Verification items for the finished model (mm, model axes). A direction names the side the tool comes from. Round coordinates to 2 decimals unless told otherwise and drop trailing zeros. Write each loop counter-clockwise with the first axis right and the second up, starting at its lowest first coordinate (ties: lowest second). Pieces come first, ordered by that corner, then holes.
from build123d import *

# Parameters (mm, degrees)
SKETCH1_W           = 16
SKETCH1_H           = 32
SKETCH1_R           = 1.5
SKETCH1_W_2         = 8
SKETCH1_H_2         = 150
BOSS_EXTRUDE1_DEPTH = 6.35
FILLET1_R           = 10
FILLET2_R           = 10
CHAMFER1_SIZE       = 10
SKETCH2_R           = 1.65
CUT_EXTRUDE1_DEPTH  = 10


with BuildPart() as part:
    # Sketch1 → Boss-Extrude1 (new body)
    # profile 1 of 3: a face of its own
    with BuildSketch(Plane.XY):
        Rectangle(SKETCH1_W, SKETCH1_H)
        with Locations((0, -8)):
            Circle(SKETCH1_R, mode=Mode.SUBTRACT)
        with Locations((0, 8)):
            Circle(SKETCH1_R, mode=Mode.SUBTRACT)
        Circle(SKETCH1_R, mode=Mode.SUBTRACT)
    # profile 2 of 3: a face of its own
    with BuildSketch(Plane.XY):
        with Locations((-4, 91)):
            Rectangle(SKETCH1_W_2, SKETCH1_H_2)
    # profile 3 of 3: a face of its own
    with BuildSketch(Plane.XY):
        Polygon((-23, -16), (-23, 166), (-8, 166), (-8, 16), (-8, -16), align=None)
    extrude(amount=BOSS_EXTRUDE1_DEPTH)

    # Fillet1
    # the kernel refuses this fillet: 10 mm, written as the material it adds along each edge
    with BuildSketch(Plane(origin=(0, 16, 0), x_dir=(0, 1, 0), z_dir=(0, 0, 1))) as fillet1_piece_1:
        with BuildLine():
            CenterArc((9.797958971, -10), FILLET1_R, 90, 78.463040967)
            Line((0, -8), (0, 0))
            Line((0, 0), (9.797958971, 0))
        make_face()
    extrude(amount=6.35)
    # the kernel refuses this fillet: 10 mm, written as the material it takes off along each edge
    with BuildSketch(Plane(origin=(8, -16, -25), x_dir=(0, 1, 0), z_dir=(0, 0, 1)), Plane(origin=(-23, -16, -25), x_dir=(1, 0, 0), z_dir=(0, 0, 1))) as fillet1_2_piece_1:
        with BuildLine():
            CenterArc((FILLET1_R, FILLET1_R), FILLET1_R, 180, 90)
            Line((0, FILLET1_R), (0, 0))
            Line((0, 0), (FILLET1_R, 0))
        make_face()
    extrude(amount=56.35, mode=Mode.SUBTRACT)

    # Fillet2
    fillet2_edges = [part.edges().sort_by_distance(p)[0] for p in [
        (8, 16, 3.175),
    ]]
    fillet(fillet2_edges, radius=FILLET2_R)

    # Chamfer1
    chamfer1_edges = [part.edges().sort_by_distance(p)[0] for p in [
        (-23, 166, 3.175),
    ]]
    chamfer(chamfer1_edges, length=CHAMFER1_SIZE)

    # Sketch2 → Cut-Extrude1 (cut)
    with BuildSketch(Plane.XY.offset(6.35)):
        with Locations((-13, 156)):
            Circle(SKETCH2_R)
        with Locations((-13, 106)):
            Circle(SKETCH2_R)
    extrude(amount=-CUT_EXTRUDE1_DEPTH, mode=Mode.SUBTRACT)


solid = part.part
Q1. Material ranges on line 1 along Y through (x, z) = (-13, 4.25); line 2 along X through (y, z) = (145, 0.5); line 3 along Y through (x, z) = (-17.5, 3), recorded low to high.
Recorded:
line 1: y = -16 to 104.35, 107.65 to 154.35, 157.65 to 166
line 2: x = -23 to 0
line 3: y = -14.93 to 161.5
Q2. Sectioned sample at B-B (z = 3.75). Enter the section's corners in (x, y), plus the area to 3 significant figures.
Recorded:
outline: (-23, -6) arc R10 ccw to (-13, -16) - (-2, -16) arc R10 ccw to (8, -6) - (8, 9.8) arc R10 ccw to (4, 17.8) arc R10 cw to (0, 25.8) - (0, 166) - (-13, 166) - (-23, 156) - close; hole circle Ø3.3 at (-13, 106); hole circle Ø3.3 at (-13, 156); hole circle Ø3 at (0, -8); hole circle Ø3 at (0, 0); hole circle Ø3 at (0, 8)
area: 4,330 mm2
Q3. Tool access check on faces 1 (the flat face through (0, 95, 3)), 2 (the cylindrical face through (4.99, -13.15, 3.13)). Record the directions out of +Z, -Z, +X, -X, +Y, -Y that give a thin tool (end or side, any length) a straight path to the whole face; none if there is none.
Recorded:
face 1: +Z, -Z, +X, +Y
face 2: +Z, -Z, +X, -Y
Q4. Depth check by flat-ended pin: P1, Ø2.5, axis at x = 0, y = 8, coming from the +Z side; P2, Ø3, axis at y = 70, z = 2.5, coming from the +X side; P3, Ø1, axis at x = -17, z = 3.5, coming from the +Y side. Enter the tip coordinate at first touch or a pass-through.
Recorded:
P1: passes through
P2: stops at x = 0
P3: stops at y = 162.5
Q5. Sectioned sample at C-C (y = 106). Enter the section's corners in (x, z).
Recorded:
outline: (-23, 0) - (-14.65, 0) - (-14.65, 6.35) - (-23, 6.35) - close; (-11.35, 0) - (0, 0) - (0, 6.35) - (-11.35, 6.35) - close
Q6. Sectioned sample at D-D (x = -17). Enter the section's corners in (y, z).
Recorded:
outline: (-15.17, 0) - (162, 0) - (162, 6.35) - (-15.17, 6.35) - close
Q7. Release check for a two-part mould opening along Y. For faces 3 (the flat face through (-7, -16, 3)), 4 (the cylindrical face through (-1.5, 0.07, 3.13)), 5 (the cylindrical face through (-12.239, 154.536, 3.219)), 6 (the flat face through (8, 2, 3)) record: released by +Y, released by -Y, zero draft, split by the parting line, or undercut.
Recorded:
face 3: released by -Y
face 4: undercut
face 5: undercut
face 6: zero draft
Q8. Sectioned sample at A-A (y = 8). Enter the section's corners in (x, z), plus the area to 3 significant figures.
Recorded:
outline: (-23, 0) - (-1.5, 0) - (-1.5, 6.35) - (-23, 6.35) - close; (1.5, 0) - (8, 0) - (8, 6.35) - (1.5, 6.35) - close
area: 178 mm2
